from build123d import *

# Parameters (mm, degrees)
SKETCH_W   = 141
SKETCH_H   = 65.3
SKETCH_R   = 4.05
SKETCH_R_2 = 1.8
SKETCH_R_3 = 1.6
SKETCH_W_2 = 18
SKETCH_H_2 = 30
PAD_DEPTH  = 3


with BuildPart() as part:
    # Sketch → Pad (new body)
    with BuildSketch(Plane.XY):
        with Locations((-70.5, 32.65)):
            Rectangle(SKETCH_W, SKETCH_H)
        with Locations((-130, 16)):
            Circle(SKETCH_R, mode=Mode.SUBTRACT)
        with Locations((-11, 16)):
            Circle(SKETCH_R, mode=Mode.SUBTRACT)
        with Locations((-134, 54.3)):
            Circle(SKETCH_R_2, mode=Mode.SUBTRACT)
        with Locations((-123, 54.3)):
            Circle(SKETCH_R_2, mode=Mode.SUBTRACT)
        with Locations((-18, 54.3)):
            Circle(SKETCH_R_2, mode=Mode.SUBTRACT)
        with Locations((-7, 54.3)):
            Circle(SKETCH_R_2, mode=Mode.SUBTRACT)
        with Locations((-5, 37.3)):
            Circle(SKETCH_R_3, mode=Mode.SUBTRACT)
        with Locations((-5, 30.8)):
            Circle(SKETCH_R_3, mode=Mode.SUBTRACT)
        with Locations((-136, 37.3)):
            Circle(SKETCH_R_3, mode=Mode.SUBTRACT)
        with Locations((-136, 30.8)):
            Circle(SKETCH_R_3, mode=Mode.SUBTRACT)
        with Locations((-84, 60.3)):
            Circle(SKETCH_R_2, mode=Mode.SUBTRACT)
        with Locations((-57, 60.3)):
            Circle(SKETCH_R_2, mode=Mode.SUBTRACT)
        with Locations((-130, 5)):
            Circle(SKETCH_R_2, mode=Mode.SUBTRACT)
        with Locations((-11, 5)):
            Circle(SKETCH_R_2, mode=Mode.SUBTRACT)
        with Locations((-58, 26)):
            Rectangle(SKETCH_W_2, SKETCH_H_2, mode=Mode.SUBTRACT)
    extrude(amount=PAD_DEPTH)


solid = part.part
Could you check a few things on this model? Use its own coordinates, in mm. A direction names the side the tool comes from. Coordinates: 2 decimals unless noted, no trailing zeros. Order: outer loops, then holes, each group sorted by start corner. A loop starts at its lowest first (then second) coordinate and runs counter-clockwise, first axis right, second up. Notation, with made-up numbers: (0.5, 28) - (40.5, 28) arc R7 cw to (40.5, 32) - close; hole circle Ø8 at (70, 78.5). An arc over 180 degrees is marked (long way). Answer in a Markdown table with one row per item. Add a question column.
(1) If we section it at A-A, the plane x = -123: Please give me the cut outline in (y, z).
(2) I need wall thicknesses on L1, parallel to Y at x = -136, z = 0.8; L2, parallel to X at y = 30.5, z = 0.6; L3, parallel to Y at x = -11, z = 0.6. Which ranges of each line are inside material? Lowest first, please.
(3) If we section it at D-D, the plane z = 2.5: State how many separate pieces and enclosed holes the cut face has, then the cut area to 3 significant figures.
(4) If we section it at B-B, the plane y = 60.3: Please give me the cut outline in (x, z), then the cut area to 3 significant figures.
(5) Will this pin go through, and if not, where does the flat tip stop? pin 1 (3 mm diameter, centred on x = -18, y = 54.3, fed in from +Z).
(6) If we section it at C-C, the plane y = 25: Please give me the cut outline in (x, z), then the cut area to 3 significant figures.
(7) On a 3-axis mill with a long thin cutter (end or side, diameter ignored), from which of +Z, -Z, +X, -X, +Y, -Y can I reach the whole of each face in a straight line? I mean faces 1 (the face through (-49, 26, 1)), 2 (the face through (-71, 33, 3)). Say none if no direction works.
(8) If we mould it in two halves opening along X, with no side actions, what happens to faces 3 (the face through (-85.327, 61.517, 1.479)), 4 (the face through (-71, 33, 0)), 5 (the face through (-141, 32, 1)), 6 (the face through (-12.428, 3.905, 1.479))? For each: released by +X, released by -X, zero draft, split by the parting line, or undercut.
Results are:
| question | item | result |
|---|---|---|
| 1 | outline | (0, 0) - (52.5, 0) - (52.5, 3) - (0, 3) - close; (56.1, 0) - (65.3, 0) - (65.3, 3) - (56.1, 3) - close |
| 2 | L1 | y = 0 to 29.2, 32.4 to 35.7, 38.9 to 65.3 |
| 2 | L2 | x = -141 to -137.57, -134.43 to -67, -49 to -6.57, -3.43 to 0 |
| 2 | L3 | y = 0 to 3.2, 6.8 to 11.95, 20.05 to 65.3 |
| 3 | separate pieces | 1 |
| 3 | enclosed holes | 15 |
| 3 | area | 8,450 mm2 |
| 4 | outline | (-141, 0) - (-85.8, 0) - (-85.8, 3) - (-141, 3) - close; (-82.2, 0) - (-58.8, 0) - (-58.8, 3) - (-82.2, 3) - close; (-55.2, 0) - (0, 0) - (0, 3) - (-55.2, 3) - close |
| 4 | area | 401 mm2 |
| 5 | pin 1 | passes through |
| 6 | outline | (-141, 0) - (-67, 0) - (-67, 3) - (-141, 3) - close; (-49, 0) - (0, 0) - (0, 3) - (-49, 3) - close |
| 6 | area | 369 mm2 |
| 7 | face 1 | +Z, -Z |
| 7 | face 2 | +Z, +X, -X, +Y, -Y |
| 8 | face 3 | undercut |
| 8 | face 4 | zero draft |
| 8 | face 5 | released by -X |
| 8 | face 6 | undercut |
